Check sheet for the modelled part. Datum: model origin and axes. Units: mm. Round coordinates to 2 decimals unless told otherwise and drop trailing zeros. Write each loop counter-clockwise with the first axis right and the second up, starting at its lowest first coordinate (ties: lowest second). Pieces come first, ordered by that corner, then holes. Notation, with made-up numbers: M 9,-10.75 L 25,-10.75 A32 ccw 25,18.25 Z; hole C -7,81 d1. An arc over 180 degrees is marked long. Answer in a Markdown table with one row per item.
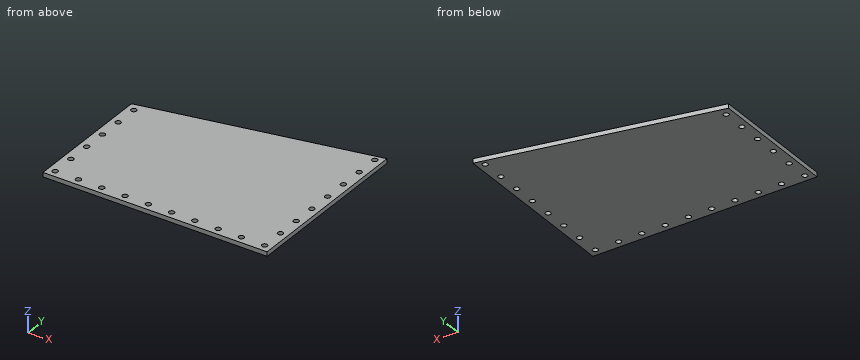
```python
from build123d import *

# Parameters (mm, degrees)
F0_R     = 1.85
F1_DEPTH = 3


with BuildPart() as f1:
    # F0 (on Top) → F1 (new body)
    with BuildSketch(Plane.XY):
        Polygon((-72, 35.5), (-72, -54.5), (82, -54.5), (82, 67.5), align=None)
        with Locations((-67, -49.5)):
            Circle(F0_R, mode=Mode.SUBTRACT)
        with Locations((-51, -49.5)):
            Circle(F0_R, mode=Mode.SUBTRACT)
        with Locations((-35, -49.5)):
            Circle(F0_R, mode=Mode.SUBTRACT)
        with Locations((-67, -33.5)):
            Circle(F0_R, mode=Mode.SUBTRACT)
        with Locations((-19, -49.5)):
            Circle(F0_R, mode=Mode.SUBTRACT)
        with Locations((-3, -49.5)):
            Circle(F0_R, mode=Mode.SUBTRACT)
        with Locations((-67, -17.5)):
            Circle(F0_R, mode=Mode.SUBTRACT)
        with Locations((-67, -1.5)):
            Circle(F0_R, mode=Mode.SUBTRACT)
        with Locations((13, -49.5)):
            Circle(F0_R, mode=Mode.SUBTRACT)
        with Locations((29, -49.5)):
            Circle(F0_R, mode=Mode.SUBTRACT)
        with Locations((45, -49.5)):
            Circle(F0_R, mode=Mode.SUBTRACT)
        with Locations((61, -49.5)):
            Circle(F0_R, mode=Mode.SUBTRACT)
        with Locations((77, -49.5)):
            Circle(F0_R, mode=Mode.SUBTRACT)
        with Locations((77, -33.5)):
            Circle(F0_R, mode=Mode.SUBTRACT)
        with Locations((77, -17.5)):
            Circle(F0_R, mode=Mode.SUBTRACT)
        with Locations((77, -1.5)):
            Circle(F0_R, mode=Mode.SUBTRACT)
        with Locations((-67, 14.5)):
            Circle(F0_R, mode=Mode.SUBTRACT)
        with Locations((-67, 30.5)):
            Circle(F0_R, mode=Mode.SUBTRACT)
        with Locations((77, 14.5)):
            Circle(F0_R, mode=Mode.SUBTRACT)
        with Locations((77, 30.5)):
            Circle(F0_R, mode=Mode.SUBTRACT)
        with Locations((77, 46.5)):
            Circle(F0_R, mode=Mode.SUBTRACT)
        with Locations((77, 62.5)):
            Circle(F0_R, mode=Mode.SUBTRACT)
    extrude(amount=F1_DEPTH)


solid = f1.part
```
1. Section check A-A, the plane y = -17.5. Record the cut outline in (x, z), and give its area (3 significant figures).
Found:
| item | result |
|---|---|
| outline | M -72,0 L -68.85,0 L -68.85,3 L -72,3 Z; M -65.15,0 L 75.15,0 L 75.15,3 L -65.15,3 Z; M 78.85,0 L 82,0 L 82,3 L 78.85,3 Z |
| area | 440 mm2 |
2. Section check D-D, the plane x = -67. Record the cut outline in (y, z), and give its area (3 significant figures).
Found:
| item | result |
|---|---|
| outline | M -54.5,0 L -51.35,0 L -51.35,3 L -54.5,3 Z; M -47.65,0 L -35.35,0 L -35.35,3 L -47.65,3 Z; M -31.65,0 L -19.35,0 L -19.35,3 L -31.65,3 Z; M -15.65,0 L -3.35,0 L -3.35,3 L -15.65,3 Z; M 0.35,0 L 12.65,0 L 12.65,3 L 0.35,3 Z; M 16.35,0 L 28.65,0 L 28.65,3 L 16.35,3 Z; M 32.35,0 L 36.54,0 L 36.54,3 L 32.35,3 Z |
| area | 207 mm2 |
3. Section check C-C, the plane y = -49.5. Count the separate pieces of the cut face and the enclosed holes in it, and give its area (3 significant figures).
Found:
| item | result |
|---|---|
| separate pieces | 11 |
| enclosed holes | 0 |
| area | 351 mm2 |
4. Go/stop test with a flat-tipped pin: pin 1 (4.5 mm diameter, centred on x = 77, y = 14.5, fed in from +Z). Record where the tip stops, or that it passes through.
Found:
| item | result |
|---|---|
| pin 1 | stops at z = 3 |
5. Section check B-B, the plane x = -35. Record the cut outline in (y, z), and give its area (3 significant figures).
Found:
| item | result |
|---|---|
| outline | M -54.5,0 L -51.35,0 L -51.35,3 L -54.5,3 Z; M -47.65,0 L 43.19,0 L 43.19,3 L -47.65,3 Z |
| area | 282 mm2 |
6. Scan lines: L1, parallel to X at y = -35, z = 1.55; L2, parallel to Y at x = 30, z = 2.5; L3, parallel to Y at x = 29, z = 1.8. Record each from-to range of solid material in increasing order.
Found:
| item | result |
|---|---|
| L1 | x = -72 to -68.08, -65.92 to 75.92, 78.08 to 82 |
| L2 | y = -54.5 to -51.06, -47.94 to 56.69 |
| L3 | y = -54.5 to -51.35, -47.65 to 56.49 |
